```python
from build123d import *

# Parameters (mm, degrees)
BOSS_EXTRUDE1_DEPTH = 50.8
SKETCH2_R           = 2.4892
CUT_EXTRUDE1_DEPTH  = 77.2
SKETCH3_R           = 2.4892
CUT_EXTRUDE2_DEPTH  = 77.2


with BuildPart() as part:
    # Sketch1 → Boss-Extrude1 (new body)
    with BuildSketch(Plane.XY):
        Polygon((0, 0), (0, 50.8), (3.175, 50.8), (3.175, 3.175), (25.4, 3.175), (25.4, 0), align=None)
    extrude(amount=BOSS_EXTRUDE1_DEPTH)

    # Sketch2 → Cut-Extrude1 (cut, through all)
    with BuildSketch(Plane(origin=(0, 0, 0), x_dir=(0, 0, -1), z_dir=(1, 0, 0))):
        with Locations(Location((-26.9875, 28.575, 0), (0, 0, 270))):
            Circle(SKETCH2_R)
    extrude(amount=CUT_EXTRUDE1_DEPTH, mode=Mode.SUBTRACT)

    # Sketch3 → Cut-Extrude2 (cut, through all)
    with BuildSketch(Plane(origin=(0, 0, 0), x_dir=(1, 0, 0), z_dir=(0, 1, 0))):
        with Locations(Location((14.2875, -38.1, 0), (0, 0, 90))):
            Circle(SKETCH3_R)
        with Locations(Location((14.2875, -12.7, 0), (0, 0, 90))):
            Circle(SKETCH3_R)
    extrude(amount=CUT_EXTRUDE2_DEPTH, mode=Mode.SUBTRACT)


solid = part.part
```
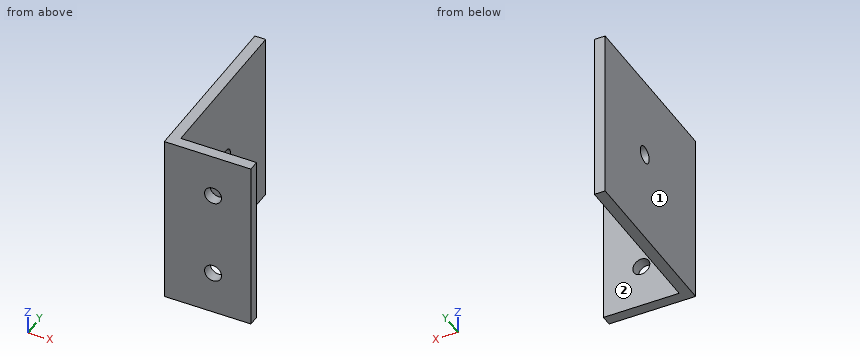
Source: CAD feature listing. Evaluate the final solid. Frame: model axes, mm. Face numbers are marked on the shaded views. A direction names the side the tool comes from. Give positions to 0.01 mm unless a question says otherwise; leave off trailing zeros. Loops run counter-clockwise (first coordinate to the right, second up) from the corner with the lowest first, then second, coordinate; pieces in that order, holes last. Notation, with made-up numbers: (-34, -11) -> (5, -11) arc R24 cw to (5, 9) -> close; hole circle Ø7 at (88, -20). An arc over 180 degrees is marked (long way). Use a Markdown table: item, result. Add a question column.
(1) Section query C-C (x = 5). Output: boundary loops of the cut face in (y, z) (3 decimals), then the cut area to 3 significant figures.
(2) First-contact query: pin 1 Ø5.5 at (y, z) = (28.58, 26.99) entering from +X (3 decimals); pin 2 Ø5 at (x, z) = (14.5, 19) entering from +Y (3 decimals). Flat tips, straight axial feed; report the tip coordinate or a pass-through.
(3) Section query A-A (z = 38.1). Output: boundary loops of the cut face in (x, y) (3 decimals).
(4) Ray query, line 1 (X direction, y = 2, z = 38); line 2 (X direction, y = 17, z = 32) (3 decimals). Return the intervals inside material, ascending.
(5) Section query D-D (z = 8.5). Output: boundary loops of the cut face in (x, y) (3 decimals), then the cut area to 3 significant figures.
(6) Section query B-B (x = 15). Output: boundary loops of the cut face in (y, z) (3 decimals), then the cut area to 3 significant figures.
(7) Access query for the marked faces 1 and 2. Directions: +Z, -Z, +X, -X, +Y, -Y. A direction counts if a zero-diameter tool reaches every point of the face in a straight line with its end or side. Return the directions, or none.
Checked values:
| question | item | result |
|---|---|---|
| 1 | outline | (0, 0) -> (3.175, 0) -> (3.175, 50.8) -> (0, 50.8) -> close |
| 1 | area | 161 mm^2 |
| 2 | pin 1 | x = 3.175 |
| 2 | pin 2 | y = 3.175 |
| 3 | outline | (0, 0) -> (11.798, 0) -> (11.798, 3.175) -> (3.175, 3.175) -> (3.175, 50.8) -> (0, 50.8) -> close; (16.777, 0) -> (25.4, 0) -> (25.4, 3.175) -> (16.777, 3.175) -> close |
| 4 | line 1 | 0 to 11.8, 16.77 to 25.4 |
| 4 | line 2 | 0 to 3.175 |
| 5 | outline | (0, 0) -> (25.4, 0) -> (25.4, 3.175) -> (3.175, 3.175) -> (3.175, 50.8) -> (0, 50.8) -> close |
| 5 | area | 232 mm^2 |
| 6 | outline | (0, 0) -> (3.175, 0) -> (3.175, 10.315) -> (0, 10.315) -> close; (0, 15.085) -> (3.175, 15.085) -> (3.175, 35.715) -> (0, 35.715) -> close; (0, 40.485) -> (3.175, 40.485) -> (3.175, 50.8) -> (0, 50.8) -> close |
| 6 | area | 131 mm^2 |
| 7 | face 1 | +Z, -Z, -X, +Y, -Y |
| 7 | face 2 | +Z, -Z, +X, +Y |
